The listing builds one solid part. Answer for the finished solid, in the listing's coordinates (mm). Face numbers are marked on the shaded views. Give positions to 0.01 mm unless a question says otherwise; leave off trailing zeros. Write each loop counter-clockwise with the first axis right and the second up, starting at its lowest first coordinate (ties: lowest second). Pieces come first, ordered by that corner, then holes. Notation, with made-up numbers: (-10, 3.25) - (-5, 3.25) arc R8 ccw to (-5, 18.25) - close; hole circle Ø8 at (34, 4.25). An arc over 180 degrees is marked (long way). Use a Markdown table: item, result. Add a question column.
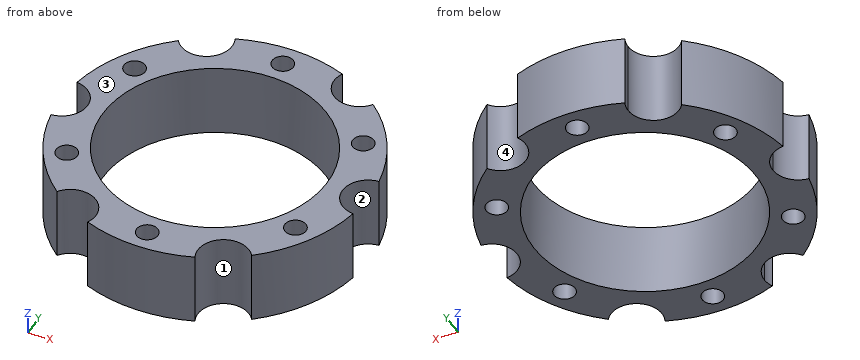
from build123d import *

# Parameters (mm, degrees)
F0_R     = 3.175
F0_R_2   = 33.3375
F1_DEPTH = 22.225


with BuildPart() as f1:
    # F0 (on Top) → F1 (new body)
    with BuildSketch(Plane.XY):
        with BuildLine():
            ThreePointArc((45.406879, -7.593861), (38.4175, 0), (45.406879, 7.593861))
            ThreePointArc((45.406879, 7.593861), (39.869645, 23.01875), (29.279916, 35.526581))
            ThreePointArc((29.279916, 35.526581), (19.20875, 33.270531), (16.126964, 43.120441))
            ThreePointArc((16.126964, 43.120441), (0, 46.0375), (-16.126964, 43.120441))
            ThreePointArc((-16.126964, 43.120441), (-15.583032, 41.535326), (-15.39875, 39.869645))
            ThreePointArc((-15.39875, 39.869645), (-20.743413, 32.597283), (-29.279916, 35.526581))
            ThreePointArc((-29.279916, 35.526581), (-39.869645, 23.01875), (-45.406879, 7.593861))
            ThreePointArc((-45.406879, 7.593861), (-40.43082, 5.160381), (-38.4175, 0))
            ThreePointArc((-38.4175, 0), (-40.43082, -5.160381), (-45.406879, -7.593861))
            ThreePointArc((-45.406879, -7.593861), (-39.869645, -23.01875), (-29.279916, -35.526581))
            ThreePointArc((-29.279916, -35.526581), (-20.743413, -32.597283), (-15.39875, -39.869645))
            ThreePointArc((-15.39875, -39.869645), (-15.583032, -41.535326), (-16.126964, -43.120441))
            ThreePointArc((-16.126964, -43.120441), (0, -46.0375), (16.126964, -43.120441))
            ThreePointArc((16.126964, -43.120441), (19.20875, -33.270531), (29.279916, -35.526581))
            ThreePointArc((29.279916, -35.526581), (39.869645, -23.01875), (45.406879, -7.593861))
        make_face()
        with Locations((-34.370383, -19.84375)):
            Circle(F0_R, mode=Mode.SUBTRACT)
        with Locations((0, -39.6875)):
            Circle(F0_R, mode=Mode.SUBTRACT)
        with Locations((34.370383, -19.84375)):
            Circle(F0_R, mode=Mode.SUBTRACT)
        with Locations((-34.370383, 19.84375)):
            Circle(F0_R, mode=Mode.SUBTRACT)
        Circle(F0_R_2, mode=Mode.SUBTRACT)
        with Locations((34.370383, 19.84375)):
            Circle(F0_R, mode=Mode.SUBTRACT)
        with Locations((0, 39.6875)):
            Circle(F0_R, mode=Mode.SUBTRACT)
    extrude(amount=F1_DEPTH)


solid = f1.part
1. Given P1, Ø2, axis at y = -14.5, z = 16.5, coming from the -X side; P2, Ø3, axis at x = 14, y = 31, coming from the -Z side; P3, Ø1, axis at x = -23.5, z = 11.5, coming from the -Y side; P4, Ø6, axis at x = 4.5, z = 18, coming from the -Y side, each flat-ended and moving along its own axis, determine where each tip first touches the part or whether it passes through.
2. Consider L1, parallel to Y at x = -33.5, z = 16.5; L2, parallel to Y at x = -35, z = 6; L3, parallel to X at y = 22, z = 7. Determine where each line is inside the solid, lowest interval first. Write a range as [from, to].
3. The part is cut by section C-C (z = 5.5). Count the separate pieces of the cut face and the enclosed holes in it, and give its area (3 significant figures).
4. For a pull along X with two mould halves and no side action, classify the marked faces 1, 2, 3 and 4 as released by +X, released by -X, zero draft, split by the parting line, or undercut.
5. The part is cut by section A-A (x = 0). Give the vertices of the cut face in (y, z) (1 decimal).
6. The part is cut by section B-B (x = -35). Give the vertices of the cut face in (y, z) (3 decimals).
7. The part is cut by section D-D (y = 2.5). Give the vertices of the cut face in (x, z) (3 decimals), and give its area (3 significant figures).
Check values:
| question | item | result |
|---|---|---|
| 1 | P1 | stops at x = -44.01 |
| 1 | P2 | stops at z = 0 |
| 1 | P3 | stops at y = -32.31 |
| 1 | P4 | stops at y = -46.01 |
| 2 | L1 | y = [-31.58, -22.9], [-16.79, 16.79], [22.9, 31.58] |
| 2 | L2 | y = [-29.91, -22.96], [-16.73, 16.73], [22.96, 29.91] |
| 2 | L3 | x = [-40.44, -36.7], [-32.04, -25.05], [25.05, 32.04], [36.7, 40.44] |
| 3 | separate pieces | 1 |
| 3 | enclosed holes | 7 |
| 3 | area | 2,450 mm2 |
| 4 | face 1 | undercut |
| 4 | face 2 | released by +X |
| 4 | face 3 | zero draft |
| 4 | face 4 | undercut |
| 5 | outline | (-46, 0) - (-42.9, 0) - (-42.9, 22.2) - (-46, 22.2) - close; (-36.5, 0) - (-33.3, 0) - (-33.3, 22.2) - (-36.5, 22.2) - close; (33.3, 0) - (36.5, 0) - (36.5, 22.2) - (33.3, 22.2) - close; (42.9, 0) - (46, 0) - (46, 22.2) - (42.9, 22.2) - close |
| 6 | outline | (-29.907, 0) - (-22.956, 0) - (-22.956, 22.225) - (-29.907, 22.225) - close; (-16.732, 0) - (16.732, 0) - (16.732, 22.225) - (-16.732, 22.225) - close; (22.956, 0) - (29.907, 0) - (29.907, 22.225) - (22.956, 22.225) - close |
| 7 | outline | (-38.839, 0) - (-33.244, 0) - (-33.244, 22.225) - (-38.839, 22.225) - close; (33.244, 0) - (38.839, 0) - (38.839, 22.225) - (33.244, 22.225) - close |
| 7 | area | 249 mm2 |
